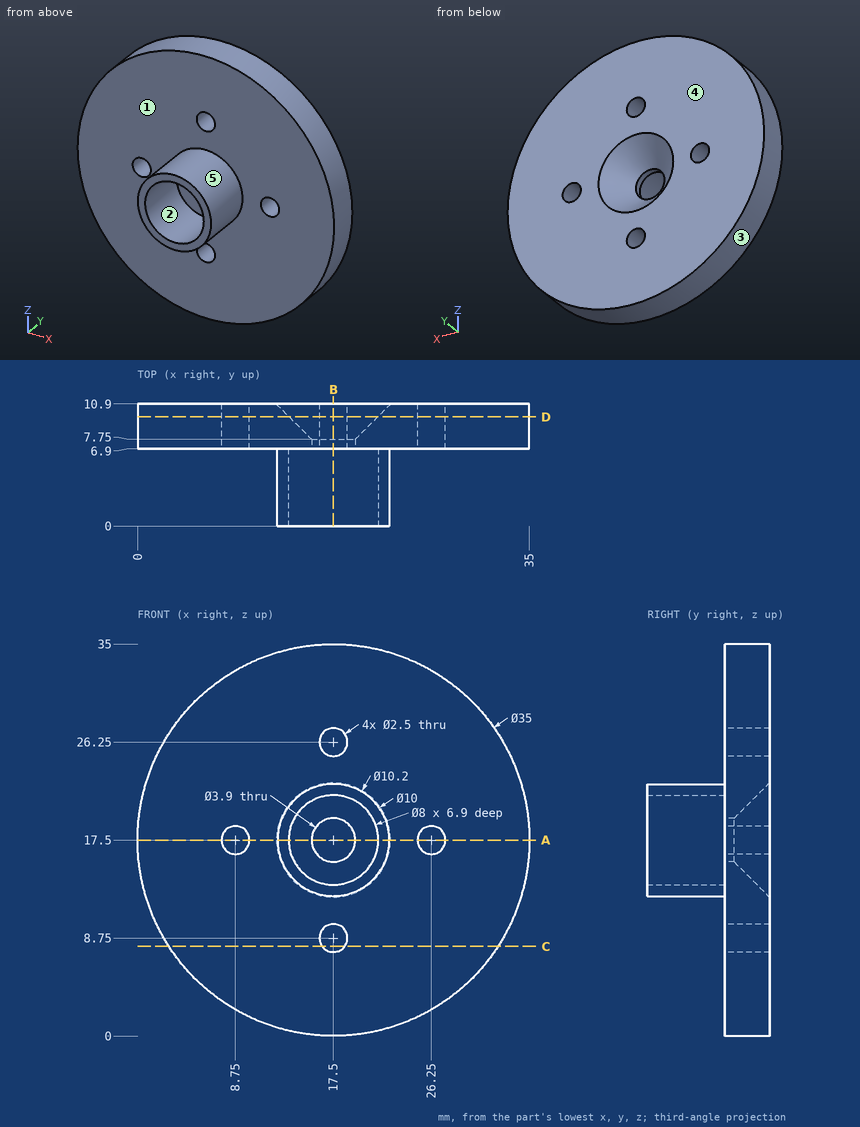
Job drawing, mm, ordinate dimensions from the low corner. One solid piece. A direction names the side the tool comes from. Give positions to 0.01 mm unless a question says otherwise; leave off trailing zeros. Order: outer loops, then holes, each group sorted by start corner. A loop starts at its lowest first (then second) coordinate and runs counter-clockwise, first axis right, second up. Notation, with made-up numbers: M -28,57.25 L 22,57.25 A9 cw 22,67.25 Z; hole C 31.25,30.25 d11. An arc over 180 degrees is marked long. Put each result on its own line as item: value. Start each with the question number.
(1) Band-saw the part on D-D on y = 9.75. Give the cut face in (x, z).
(2) Band-saw the part on B-B on x = 17.5. Give the cut face in (y, z).
(3) Pull direction Z, two halves, no side cores. Call the marked faces 1, 2 and 3: released by +Z, released by -Z, zero draft, split by the parting line, or undercut.
(4) Band-saw the part on C-C on z = 8. Give the cut face in (x, y), then the cut area to 3 significant figures.
(5) Tool access for the marked faces 4 and 5: list every direction of +Z, -Z, +X, -X, +Y, -Y with a clear straight run to the whole face (end or side of a thin tool).
(6) Pin check, flat tips, straight feed: pin 1 Ø1.5 at (x, z) = (17.5, 8.75) entering from -Y; pin 2 Ø4 at (y, z) = (8, 20) entering from -X; pin 3 Ø3 at (x, z) = (14.5, 18.5) entering from -Y; pin 4 Ø3 at (x, z) = (26.25, 17.5) entering from -Y. Stop position of each tip, or through.
(7) Drill centre lines: L1, parallel to Z at x = 17.5, y = 7.3; L2, parallel to Z at x = 17.5, y = 8.65; L3, parallel to Z at x = 17.5, y = 1.5. Where is each one in solid material? Low to high. Write a range as [from, to].
(8) Band-saw the part on A-A on z = 17.5. Give the cut face in (x, y).
Results below:
1. outline: C 17.5,17.5 d35; hole C 8.75,17.5 d2.5; hole C 17.5,17.5 d7.9; hole C 17.5,8.75 d2.5; hole C 17.5,26.25 d2.5; hole C 26.25,17.5 d2.5
2. outline: M 0,12.5 L 6.9,12.5 L 6.9,10 L 10.9,10 L 10.9,12.4 L 7.75,15.55 L 6.9,15.55 L 6.9,13.5 L 0,13.5 Z; M 0,21.5 L 6.9,21.5 L 6.9,19.45 L 7.75,19.45 L 10.9,22.6 L 10.9,25 L 6.9,25 L 6.9,22.5 L 0,22.5 Z; M 6.9,0 L 10.9,0 L 10.9,7.5 L 6.9,7.5 Z; M 6.9,27.5 L 10.9,27.5 L 10.9,35 L 6.9,35 Z
3. face 1: zero draft
3. face 2: undercut
3. face 3: split by the parting line
4. outline: M 2.8,6.9 L 16.5,6.9 L 16.5,10.9 L 2.8,10.9 Z; M 18.5,6.9 L 32.2,6.9 L 32.2,10.9 L 18.5,10.9 Z
4. area: 110 mm2
5. face 4: +Z, -Z, +X, -X, +Y
5. face 5: -Y
6. pin 1: passes through
6. pin 2: stops at x = 0.01
6. pin 3: stops at y = 0
6. pin 4: stops at y = 6.9
7. L1: z = [0, 7.5], [10, 15.55], [19.45, 25], [27.5, 35]
7. L2: z = [0, 7.5], [10, 14.65], [20.35, 25], [27.5, 35]
7. L3: z = [12.5, 13.5], [21.5, 22.5]
8. outline: M 0,6.9 L 7.5,6.9 L 7.5,10.9 L 0,10.9 Z; M 10,6.9 L 12.5,6.9 L 12.5,0 L 13.5,0 L 13.5,6.9 L 15.55,6.9 L 15.55,7.75 L 12.4,10.9 L 10,10.9 Z; M 19.45,6.9 L 21.5,6.9 L 21.5,0 L 22.5,0 L 22.5,6.9 L 25,6.9 L 25,10.9 L 22.6,10.9 L 19.45,7.75 Z; M 27.5,6.9 L 35,6.9 L 35,10.9 L 27.5,10.9 Z
